Source: CAD feature listing. Evaluate the final solid. Frame: model axes, mm. A direction names the side the tool comes from. Give positions to 0.01 mm unless a question says otherwise; leave off trailing zeros. Order: outer loops, then holes, each group sorted by start corner. A loop starts at its lowest first (then second) coordinate and runs counter-clockwise, first axis right, second up. Notation, with made-up numbers: (-28, 32.25) - (2, 32.25) arc R9 cw to (2, 40.25) - close; hole circle Ø7 at (36, 17). An arc over 180 degrees is marked (long way). Write each question's results on one line, items separated by ' | '. Start each with the question number.
Item 1: Line query: line 1 along Y through (x, z) = (-129, -0.75); line 2 along X through (y, z) = (36, 5.25); line 3 along X through (y, z) = (93.5, -1.75). Output: solid intervals per line, ascending.
Item 2: Section C-C on y = 69.5. Output: boundary loops of the cut face in (x, z).
Item 3: Section A-A on y = 0. Output: boundary loops of the cut face in (x, z).
Item 4: Mould query, pull axis X, two halves, no side actions, for faces 1 (the flat face through (-240.442, 46, 0)), 2 (the flat face through (60, 149.184, 0)), 3 (the cylindrical face through (-227.083, 46.689, -0.089)). Classes: released by +X, released by -X, zero draft, split by the parting line, or undercut.
Item 5: Section B-B on x = -179. Output: boundary loops of the cut face in (y, z), and give its area (3 significant figures).
Item 6: Contact query for a flat-ended pin moving along its axis: pin 1 Ø11.5 at (x, y) = (355.3, 49.35) entering from -Z (3 decimals). Output: stop coordinate, or through.
Item 7: Section D-D on z = 2.5. Output: boundary loops of the cut face in (x, y), and give its area (3 significant figures).
Item 8: Set-up query: faces 4 (the flat face through (67, 136.484, 0)), 5 (the flat face through (369.158, 46, 0)). Return all of +Z, -Z, +X, -X, +Y, -Y with unobstructed straight access to the full face (end or side cutting, diameter ignored); none if empty.
```python
from build123d import *

# Parameters (mm, degrees)
F0_W     = 609.6
F0_H     = 203.2
F0_W_2   = 546.1
F0_H_2   = 177.8
F1_DEPTH = 6.35
F3_D     = 12.7
F5_D     = 12.7


with BuildPart() as f1:
    # F0 (on Top) → F1 (new body, symmetric)
    with BuildSketch(Plane.XY):
        with Locations((64.358067, 47.583953)):
            Rectangle(F0_W, F0_H)
        with Locations((70.708067, 47.583953)):
            Rectangle(F0_W_2, F0_H_2, mode=Mode.SUBTRACT)
    extrude(amount=F1_DEPTH, both=True)

    # F3 (through all)
    with Locations(Plane.XY.offset(6.35)):
        with Locations((-221.025839, 99.038169), (-221.025839, 44.781234), (-220.216036, 0)):
            Hole(F3_D / 2)

    # F5 (through all)
    with Locations(Plane.XY.offset(6.35)):
        with Locations((355.980128, 104.1537), (355.303496, 49.347699), (354.626894, 0)):
            Hole(F5_D / 2)


solid = f1.part
```
Evaluation:
1) line 1: y = -54.02 to -41.32, 136.48 to 149.18 | line 2: x = -240.44 to -202.34, 343.76 to 369.16 | line 3: x = -240.44 to -224.13, -217.92 to -202.34, 343.76 to 369.16
2) outline: (-240.44, -6.35) - (-202.34, -6.35) - (-202.34, 6.35) - (-240.44, 6.35) - close; (343.76, -6.35) - (369.16, -6.35) - (369.16, 6.35) - (343.76, 6.35) - close
3) outline: (-240.44, -6.35) - (-226.57, -6.35) - (-226.57, 6.35) - (-240.44, 6.35) - close; (-213.87, -6.35) - (-202.34, -6.35) - (-202.34, 6.35) - (-213.87, 6.35) - close; (343.76, -6.35) - (348.28, -6.35) - (348.28, 6.35) - (343.76, 6.35) - close; (360.98, -6.35) - (369.16, -6.35) - (369.16, 6.35) - (360.98, 6.35) - close
4) face 1: released by -X | face 2: zero draft | face 3: undercut
5) outline: (-54.02, -6.35) - (-41.32, -6.35) - (-41.32, 6.35) - (-54.02, 6.35) - close; (136.48, -6.35) - (149.18, -6.35) - (149.18, 6.35) - (136.48, 6.35) - close | area: 323 mm^2
6) pin 1: passes through
7) outline: (-240.44, -54.02) - (369.16, -54.02) - (369.16, 149.18) - (-240.44, 149.18) - close; hole circle Ø12.7 at (-221.03, 44.78); hole circle Ø12.7 at (-221.03, 99.04); hole circle Ø12.7 at (-220.22, 0); hole (-202.34, -41.32) - (343.76, -41.32) - (343.76, 136.48) - (-202.34, 136.48) - close; hole circle Ø12.7 at (354.63, 0); hole circle Ø12.7 at (355.3, 49.35); hole circle Ø12.7 at (355.98, 104.15) | area: 26,000 mm^2
8) face 4: +Z, -Z | face 5: +Z, -Z, +X, +Y, -Y
